from build123d import *

# Parameters (mm, degrees)
SKETCH1_R           = 7
BOSS_EXTRUDE1_DEPTH = 15
SKETCH2_R           = 3.75
BOSS_EXTRUDE2_DEPTH = 7
SKETCH3_R           = 1.75
CUT_EXTRUDE1_DEPTH  = 22


with BuildPart() as part:
    # Sketch1 → Boss-Extrude1 (new body)
    with BuildSketch(Plane(origin=(0, 0, 0), x_dir=(0, 1, 0), z_dir=(0, 0, 1))):
        with Locations(Location((0, 0, 0), (0, 0, 270))):
            Circle(SKETCH1_R)
    extrude(amount=BOSS_EXTRUDE1_DEPTH)

    # Sketch2 → Boss-Extrude2 (add)
    with BuildSketch(Plane.XY.offset(15)):
        Circle(SKETCH2_R)
    extrude(amount=BOSS_EXTRUDE2_DEPTH)

    # Sketch3 → Cut-Extrude1 (cut)
    with BuildSketch(Plane.XY.offset(22)):
        Circle(SKETCH3_R)
    extrude(amount=-CUT_EXTRUDE1_DEPTH, mode=Mode.SUBTRACT)


solid = part.part
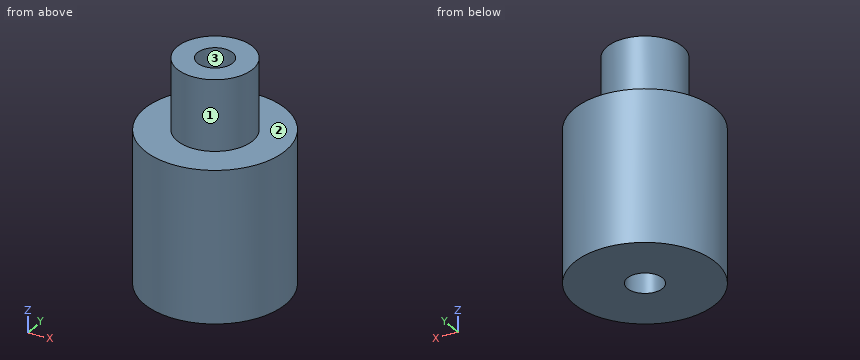
Verification items for the finished model (mm, model axes). Face numbers are marked on the shaded views. Give positions to 0.01 mm unless a question says otherwise; leave off trailing zeros. Order: outer loops, then holes, each group sorted by start corner. A loop starts at its lowest first (then second) coordinate and runs counter-clockwise, first axis right, second up. Notation, with made-up numbers: M 70.25,14.5 L 118.25,14.5 A22 cw 118.25,24.5 Z; hole C 13,2 d2. An arc over 180 degrees is marked long. Answer as a JSON object with one key per item and string values. Group by question number.
1) Depth check by flat-ended pin: pin 1 Ø1 at (y, z) = (3, 7.5) entering from +X; pin 2 Ø2 at (x, z) = (-3.5, 18) entering from -Y; pin 3 Ø1.5 at (x, z) = (-1.5, 14) entering from +Y. Enter the tip coordinate at first touch or a pass-through.
2) Scan lines: line 1 along Y through (x, z) = (0, 10.75); line 2 along Y through (x, z) = (0, 15.5); line 3 along Z through (x, y) = (-5.75, -1.25). Record each from-to range of solid material in increasing order. Write a range as [from, to].
3) Cross-section at A-A (y = 0). Enter the section's corners in (x, z).
4) Cross-section at D-D (y = 2.75). Enter the section's corners in (x, z), then the cut area to 3 significant figures.
5) Mould release check, pull along X, two halves, no side actions. Record for the marked faces 1, 2 and 3: released by +X, released by -X, zero draft, split by the parting line, or undercut.
6) Cross-section at C-C (z = 2). Enter the section's corners in (x, y).
Result sheet:
{
 "1": {"pin 1": "stops at x = 6.54", "pin 2": "stops at y = -2.8", "pin 3": "stops at y = 6.96"},
 "2": {"line 1": "y = [-7, -1.75], [1.75, 7]", "line 2": "y = [-3.75, -1.75], [1.75, 3.75]", "line 3": "z = [0, 15]"},
 "3": {"outline": "M -7,0 L -1.75,0 L -1.75,22 L -3.75,22 L -3.75,15 L -7,15 Z; M 1.75,0 L 7,0 L 7,15 L 3.75,15 L 3.75,22 L 1.75,22 Z"},
 "4": {"outline": "M -6.44,0 L 6.44,0 L 6.44,15 L 2.55,15 L 2.55,22 L -2.55,22 L -2.55,15 L -6.44,15 Z", "area": "229 mm2"},
 "5": {"face 1": "split by the parting line", "face 2": "zero draft", "face 3": "undercut"},
 "6": {"outline": "C 0,0 d14; hole C 0,0 d3.5"}
}
